Verification items for this drawing (mm, ordinates from the low corner). A direction names the side the tool comes from. Coordinates: 2 decimals unless noted, no trailing zeros. Loops run counter-clockwise (first coordinate to the right, second up) from the corner with the lowest first, then second, coordinate; pieces in that order, holes last. Notation, with made-up numbers: M 70,-37.75 L 111,-37.75 A27 ccw 111,-11.75 Z; hole C 50.5,27.5 d4. An arc over 180 degrees is marked long. Use CSV: the item, a comma, the result in double quotes.
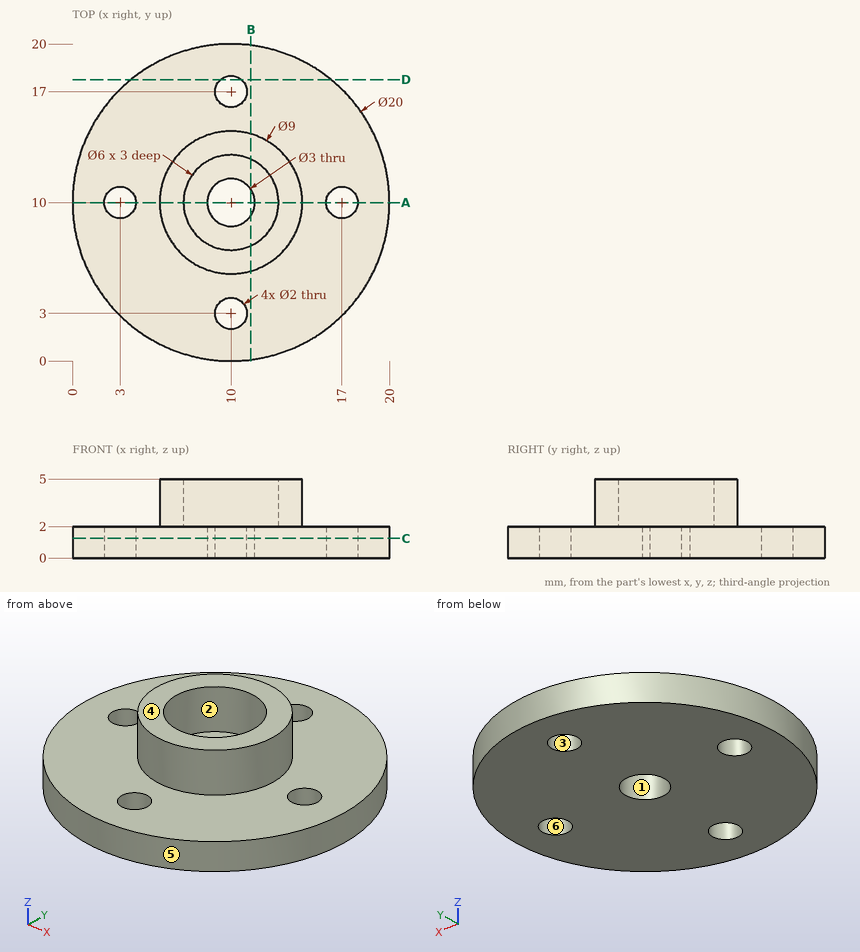
1. Section check B-B, the plane x = 11.25. Record the cut outline in (y, z), plus the area to 3 significant figures.
The answers:
outline,"M 0.08,0 L 9.17,0 L 9.17,2 L 7.27,2 L 7.27,5 L 5.68,5 L 5.68,2 L 0.08,2 Z; M 10.83,0 L 19.92,0 L 19.92,2 L 14.32,2 L 14.32,5 L 12.73,5 L 12.73,2 L 10.83,2 Z"
area,"45.9 mm^2"
2. Section check A-A, the plane y = 10. Record the cut outline in (x, z), plus the area to 3 significant figures.
The answers:
outline,"M 0,0 L 2,0 L 2,2 L 0,2 Z; M 4,0 L 8.5,0 L 8.5,2 L 7,2 L 7,5 L 5.5,5 L 5.5,2 L 4,2 Z; M 11.5,0 L 16,0 L 16,2 L 14.5,2 L 14.5,5 L 13,5 L 13,2 L 11.5,2 Z; M 18,0 L 20,0 L 20,2 L 18,2 Z"
area,"35.0 mm^2"
3. Thickness scan on line 1 (Y direction, x = 10, z = 0.9); line 2 (Z direction, x = 4.5, y = 15.5); line 3 (Y direction, x = 10.25, z = 3). Record the ranges inside material, lowest first. Write a range as [from, to].
The answers:
line 1,"[0, 2], [4, 8.5], [11.5, 16], [18, 20]"
line 2,"[0, 2]"
line 3,"[5.51, 7.01], [12.99, 14.49]"
4. Gauge pin test, flat ends, axial feed: P1, Ø12, axis at x = 9, y = 3, coming from the -Z side; P2, Ø4, axis at x = 11.5, y = 17.5, coming from the +Z side; P3, Ø2, axis at y = 8, z = 2, coming from the +X side. Record the tip position at first contact, or that the pin passes through.
The answers:
P1,"z = 0"
P2,"z = 2"
P3,"x = 19.95"
5. Section check C-C, the plane z = 1.25. Record the cut outline in (x, y).
The answers:
outline,"C 10,10 d20; hole C 3,10 d2; hole C 10,10 d3; hole C 10,3 d2; hole C 10,17 d2; hole C 17,10 d2"
6. Section check D-D, the plane y = 17.75. Record the cut outline in (x, z), plus the area to 3 significant figures.
The answers:
outline,"M 3.68,0 L 9.34,0 L 9.34,2 L 3.68,2 Z; M 10.66,0 L 16.32,0 L 16.32,2 L 10.66,2 Z"
area,"22.6 mm^2"
7. Release check for a two-part mould opening along X. For the marked faces 3, 4, 5 and 6 record: +X half, -X half, draft (parallel to the pull), parting line (faces both ways), or undercut.
The answers:
face 3,"undercut"
face 4,"draft"
face 5,"parting line"
face 6,"undercut"
8. Set-up check for the marked faces 1 and 2: record each of +Z, -Z, +X, -X, +Y, -Y from which the full face is reachable in a straight line by a thin tool's end or side.
The answers:
face 1,"+Z, -Z"
face 2,"+Z"
